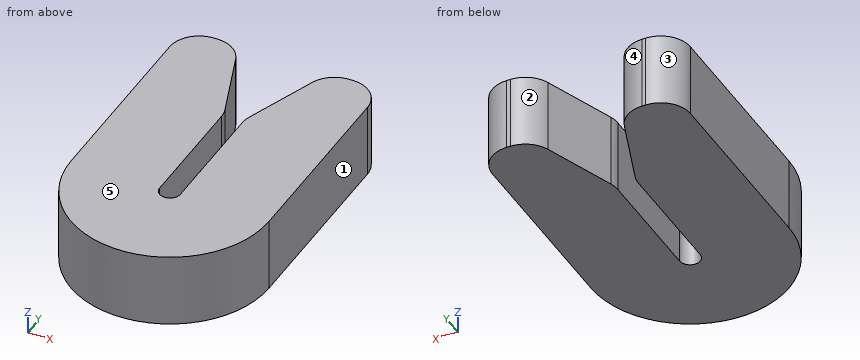
```python
from build123d import *

# Parameters (mm, degrees)
BOSS_EXTRUDE1_DEPTH = 5
FILLET2_R           = 2


with BuildPart() as part:
    # Sketch1 → Boss-Extrude1 (new body)
    with BuildSketch(Plane.XY):
        with BuildLine():
            Line((-0.7, 0), (-0.7, 8.511007364))
            Line((-0.7, 8.511007364), (-3.06180017, 15))
            Line((-3.06180017, 15), (-6.7, 15))
            Line((-6.7, 15), (-6.7, 0))
            ThreePointArc((-6.7, 0), (0, -6.7), (6.7, 0))
            Line((6.7, 0), (6.7, 15))
            Line((6.7, 15), (3.06180017, 15))
            Line((3.06180017, 15), (0.7, 8.511007364))
            Line((0.7, 8.511007364), (0.7, 0))
            ThreePointArc((0.7, 0), (0, -0.7), (-0.7, 0))
        make_face()
    extrude(amount=BOSS_EXTRUDE1_DEPTH)

    # Fillet2
    fillet2_edges = [part.edges().sort_by_distance(p)[0] for p in [
        (3.06180017, 15, 2.5),
        (6.7, 15, 2.5),
        (-6.7, 15, 2.5),
        (-3.06180017, 15, 2.5),
        (-0.7, 8.511007364, 2.5),
        (0.7, 8.511007364, 2.5),
    ]]
    fillet(fillet2_edges, radius=FILLET2_R)


solid = part.part
```
Geometry: final body of the model. Coordinates: model frame, mm. Face numbers are marked on the shaded views. A direction names the side the tool comes from. Round coordinates to 2 decimals unless told otherwise and drop trailing zeros. Loops run counter-clockwise (first coordinate to the right, second up) from the corner with the lowest first, then second, coordinate; pieces in that order, holes last. Notation, with made-up numbers: (13, 75) -> (43, 75) arc R19 cw to (43, 95) -> close; hole circle Ø6 at (54.25, -31). An arc over 180 degrees is marked (long way). Use one line per item in the form item = value. Start each with the question number.
1) Line query: L1, parallel to X at y = 6.25, z = 3.5; L2, parallel to X at y = 10, z = 2.1; L3, parallel to Y at x = 5.5, z = 0.35. Output: solid intervals per line, ascending.
2) Section C-C on y = 8.5. Output: boundary loops of the cut face in (x, z).
3) First-contact query: P1, Ø1.5, axis at x = 4.5, y = -3, coming from the -Z side; P2, Ø1, axis at y = -2.5, z = 1.5, coming from the -X side; P3, Ø1.5, axis at y = -3.5, z = 2, coming from the -X side; P4, Ø1, axis at y = -3, z = 2.5, coming from the -X side. Flat tips, straight axial feed; report the tip coordinate or a pass-through.
4) Section D-D on x = 0. Output: boundary loops of the cut face in (y, z).
5) Draft query along X for the marked faces 1, 2 and 3. Return one class per face: released by +X, released by -X, zero draft, split by the parting line, or undercut.
6) Access query for the marked faces 4 and 5. Directions: +Z, -Z, +X, -X, +Y, -Y. A direction counts if a zero-diameter tool reaches every point of the face in a straight line with its end or side. Return the directions, or none.
7) Section A-A on y = 6. Output: boundary loops of the cut face in (x, z), then the cut area to 3 significant figures.
8) Section B-B on z = 3.3. Output: boundary loops of the cut face in (x, y).
Response:
q1.L1 = -6.7 to -0.7, 0.7 to 6.7
q1.L2 = -6.7 to -1.24, 1.24 to 6.7
q1.L3 = -3.83 to 14.83
q2.outline = (-6.7, 0) -> (-0.73, 0) -> (-0.73, 5) -> (-6.7, 5) -> close; (0.73, 0) -> (6.7, 0) -> (6.7, 5) -> (0.73, 5) -> close
q3.P1 = 0
q3.P2 = -6.39
q3.P3 = -6.11
q3.P4 = -6.22
q4.outline = (-6.7, 0) -> (-0.7, 0) -> (-0.7, 5) -> (-6.7, 5) -> close
q5.face_1 = released by +X
q5.face_2 = undercut
q5.face_3 = released by -X
q6.face_4 = +Z, -Z, +Y
q6.face_5 = +Z, +X, -X, +Y, -Y
q7.outline = (-6.7, 0) -> (-0.7, 0) -> (-0.7, 5) -> (-6.7, 5) -> close; (0.7, 0) -> (6.7, 0) -> (6.7, 5) -> (0.7, 5) -> close
q7.area = 60.0 mm^2
q8.outline = (-6.7, 0) arc R6.7 ccw to (6.7, 0) -> (6.7, 13) arc R2 ccw to (4.7, 15) -> (4.46, 15) arc R2 ccw to (2.58, 13.68) -> (0.82, 8.84) arc R2 ccw to (0.7, 8.16) -> (0.7, 0) arc R0.7 cw to (-0.7, 0) -> (-0.7, 8.16) arc R2 ccw to (-0.82, 8.84) -> (-2.58, 13.68) arc R2 ccw to (-4.46, 15) -> (-4.7, 15) arc R2 ccw to (-6.7, 13) -> close
